Check sheet for the modelled part. Datum: model origin and axes. Units: mm. A direction names the side the tool comes from. Round coordinates to 2 decimals unless told otherwise and drop trailing zeros. Write each loop counter-clockwise with the first axis right and the second up, starting at its lowest first coordinate (ties: lowest second). Pieces come first, ordered by that corner, then holes. Notation, with made-up numbers: M 39.25,-22 L 43.25,-22 A12 cw 43.25,-15 Z; hole C 49,15.25 d8. An arc over 180 degrees is marked long. One line per item, written item: value.
from build123d import *

# Parameters (mm, degrees)
BOSS_EXTRUDE1_DEPTH = 4
SKETCH2_R           = 2.5
CUT_EXTRUDE1_DEPTH  = 147.546920814


with BuildPart() as part:
    # Sketch1 → Boss-Extrude1 (new body)
    with BuildSketch(Plane(origin=(0, 0, 0), x_dir=(0, 0, -1), z_dir=(1, 0, 0))):
        Polygon((0, 63), (0, 78), (124, 78), (124, 63), (110, 63), (110, 15), (124, 15), (124, 0), (0, 0), (0, 15), (-4, 15), (-4, 63), align=None)
    extrude(amount=BOSS_EXTRUDE1_DEPTH)

    # Sketch2 → Cut-Extrude1 (cut, through all)
    with BuildSketch(Plane(origin=(4, 0, 0), x_dir=(0, 0, -1), z_dir=(1, 0, 0))):
        with Locations((42, 24.5)):
            Circle(SKETCH2_R)
        with Locations((42, 53.5)):
            Circle(SKETCH2_R)
        with Locations((82.5, 53)):
            Circle(SKETCH2_R)
    extrude(amount=-CUT_EXTRUDE1_DEPTH, mode=Mode.SUBTRACT)


solid = part.part
Q1. Scan lines: line 1 (Y direction, x = 1.3, z = -42); line 2 (Z direction, x = 0.5, y = 54); line 3 (Z direction, x = 1.1, y = 4). Record each from-to range of solid material in increasing order. Write a range as [from, to].
Completed:
line 1: [0, 22], [27, 51], [56, 78]
line 2: [-110, -84.79], [-80.21, -44.45], [-39.55, 4]
line 3: [-124, 0]
Q2. Sectioned sample at B-B on x = 1.25. Enter the section's corners in (y, z).
Completed:
outline: M 0,-124 L 15,-124 L 15,-110 L 63,-110 L 63,-124 L 78,-124 L 78,0 L 63,0 L 63,4 L 15,4 L 15,0 L 0,0 Z; hole C 24.5,-42 d5; hole C 53,-82.5 d5; hole C 53.5,-42 d5
Q3. Draft check along Y on faces 5 (the flat face through (4, 40, -61)), 6 (the flat face through (2, 0, -63)), 7 (the flat face through (2, 63, -117)). Enter one of: pulls with the +Y half, pulls with the -Y half, needs draft (parallel to the pull), parting line crosses it, or undercut.
Completed:
face 5: needs draft
face 6: pulls with the -Y half
face 7: undercut
Q4. Sectioned sample at D-D on z = -42. Enter the section's corners in (x, y).
Completed:
outline: M 0,0 L 4,0 L 4,22 L 0,22 Z; M 0,27 L 4,27 L 4,51 L 0,51 Z; M 0,56 L 4,56 L 4,78 L 0,78 Z
Q5. Sectioned sample at C-C on z = -82.5. Enter the section's corners in (x, y).
Completed:
outline: M 0,0 L 4,0 L 4,50.5 L 0,50.5 Z; M 0,55.5 L 4,55.5 L 4,78 L 0,78 Z
Q6. Depth check by flat-ended pin: P1, Ø1.2, axis at x = 2.5, z = 2, coming from the +Y side; P2, Ø2, axis at x = 2, y = 5.5, coming from the +Z side. Enter the tip coordinate at first touch or a pass-through.
Completed:
P1: y = 63
P2: z = 0
Q7. Sectioned sample at A-A on y = 24.5. Enter the section's corners in (x, z), and give its area (3 significant figures).
Completed:
outline: M 0,-110 L 4,-110 L 4,-44.5 L 0,-44.5 Z; M 0,-39.5 L 4,-39.5 L 4,4 L 0,4 Z
area: 436 mm^2
Q8. Access from +Z, -Z, +X, -X, +Y, -Y to the whole of each face (thin tool, end or side, straight path). Record for faces 1 (the flat face through (2, 39, -110)), 2 (the flat face through (2, 70, 0)), 3 (the cylindrical face through (2.03, 26.61, -43.34)), 4 (the flat face through (2, 7, 0)).
Completed:
face 1: -Z, +X, -X
face 2: +Z, +X, -X, +Y
face 3: +X, -X
face 4: +Z, +X, -X, -Y
